Geometry check sheet. Reference: the model listing, model coordinates, mm. A direction names the side the tool comes from. Coordinates: 2 decimals unless noted, no trailing zeros. Write each loop counter-clockwise with the first axis right and the second up, starting at its lowest first coordinate (ties: lowest second). Pieces come first, ordered by that corner, then holes. Notation, with made-up numbers: (14.25, -36.75) -> (70.25, -36.75) arc R27 cw to (70.25, 2.25) -> close; hole circle Ø8 at (-35, 55). An arc over 180 degrees is marked (long way). One line per question, with ' | ' between items.
Autodesk Inventor part; units mm, degrees
ref_plane "YZ Plane" through (0, 0, 0) normal (1, 0, 0) x (0, 1, 0)
ref_plane "XZ Plane" through (0, 0, 0) normal (0, 1, 0) x (-1, 0, 0)
ref_plane "XY Plane" through (0, 0, 0) normal (0, 0, 1) x (1, 0, 0)
sketch "Sketch1" plane through (0, 0, 0) normal (0, 0, 1) x (1, 0, 0)
  line L0 (0, 0) -> (0, 63.8302)
  line L1 (0, 63.8302) -> (11.8288, 63.8302)
  line L2 (11.8288, 63.8302) -> (86.0806, 13.7465)
  line L3 (86.0806, 13.7465) -> (86.0806, 0)
  line L4 (86.0806, 0) -> (0, 0)
  dimension "d0" = 11.8288
  dimension "d1" = 13.7465
  dimension "d2" = 63.8302
  dimension "d3" = 86.0806
extrude "Extrusion1" add sketch "Sketch1" along normal blind 13.0607
sketch "Sketch3" plane through (0, 0, 13.0607) normal (0, 0, 1) x (1, 0, 0)
  line L0 (86.0806, 0) -> (86.0806, 13.7465)
  line L1 (86.0806, 13.7465) -> (0, 13.7465)
  line L2 (0, 13.7465) -> (0, 0)
  line L3 (0, 0) -> (86.0806, 0)
  line L4 (86.0806, 0) -> (86.0806, 13.7465)
extrude "Extrusion2" add sketch "Sketch3" along normal blind 24.1529
sketch "Sketch4" plane through (0, 0, 13.0607) normal (0, 0, 1) x (1, 0, 0)
  circle A0 centre (14.478, 33.0708) radius 7.5463
  line L0 (11.8288, 63.8302) -> (0, 63.8302)
  line L1 (0, 63.8302) -> (0, 13.7465)
  point P0 (0, 0)
  dimension "d8" = 15.0927
  dimension "d9" = 30.7594
  dimension "d10" = 14.478
extrude "Extrusion3" cut sketch "Sketch4" against normal blind 24.1529
properties part number "WoodenBlock" material "Stainless Steel"
(1) Cross-section at B-B (y = 27). Record the cut outline in (x, z), plus the area to 3 significant figures.
Answers below:
outline: (0, 0) -> (10, 0) -> (10, 13.06) -> (0, 13.06) -> close; (18.96, 0) -> (66.43, 0) -> (66.43, 13.06) -> (18.96, 13.06) -> close | area: 751 mm²
(2) Tool access check on faces 1 (the face through (33, 25, 0)), 2 (the face through (44, 13.746, 25)). Record the directions out of +Z, -Z, +X, -X, +Y, -Y that give a thin tool (end or side, any length) a straight path to the whole face; none if there is none.
Answers below:
face 1: -Z, +X, -X, +Y, -Y | face 2: +Z, +X, -X, +Y
(3) Cross-section at A-A (x = 18). Record the cut outline in (y, z), plus the area to 3 significant figures.
Answers below:
outline: (0, 0) -> (26.4, 0) -> (26.4, 13.06) -> (13.75, 13.06) -> (13.75, 37.21) -> (0, 37.21) -> close; (39.74, 0) -> (59.67, 0) -> (59.67, 13.06) -> (39.74, 13.06) -> close | area: 937 mm²
(4) Draft check along X on faces 3 (the face through (86.081, 7, 18)), 4 (the face through (13.496, 40.553, 6.622)), 5 (the face through (44, 0, 18)). Enter one of: pulls with the +X half, pulls with the -X half, needs draft (parallel to the pull), parting line crosses it, or undercut.
Answers below:
face 3: pulls with the +X half | face 4: undercut | face 5: needs draft
(5) Cross-section at C-C (z = 18). Record the cut outline in (x, y), plus the area to 3 significant figures.
Answers below:
outline: (0, 0) -> (86.08, 0) -> (86.08, 13.75) -> (0, 13.75) -> close | area: 1,180 mm²
(6) Depth check by flat-ended pin: P1, Ø3, axis at x = 66.5, y = 16, coming from the +Z side; P2, Ø1, axis at x = 52.5, z = 11.5, coming from the -Y side; P3, Ø9, axis at x = 14.48, y = 33.07, coming from the -Z side; P4, Ø6, axis at x = 69.5, z = 10, coming from the +Y side. Enter the tip coordinate at first touch or a pass-through.
Answers below:
P1: stops at z = 13.06 | P2: stops at y = 0 | P3: passes through | P4: stops at y = 26.95
(7) Material ranges on line 1 (Y direction, x = 21, z = 14.5); line 2 (Z direction, x = 8, y = 23); line 3 (X direction, y = 61.5, z = 9), recorded low to high.
Answers below:
line 1: y = 0 to 13.75 | line 2: z = 0 to 13.06 | line 3: x = 0 to 15.28
(8) Cross-section at D-D (x = 65.5). Record the cut outline in (y, z).
Answers below:
outline: (0, 0) -> (27.63, 0) -> (27.63, 13.06) -> (13.75, 13.06) -> (13.75, 37.21) -> (0, 37.21) -> close
